Geometry check sheet. Reference: the model listing, model coordinates, mm. Face numbers are marked on the shaded views. A direction names the side the tool comes from. Give positions to 0.01 mm unless a question says otherwise; leave off trailing zeros. Loops run counter-clockwise (first coordinate to the right, second up) from the corner with the lowest first, then second, coordinate; pieces in that order, holes last. Notation, with made-up numbers: (-17, 20) -> (-8, 20) arc R24 cw to (-8, 30) -> close; hole circle Ø10 at (83, -10.75). An arc over 180 degrees is marked (long way). One line per question, with ' | ' between items.
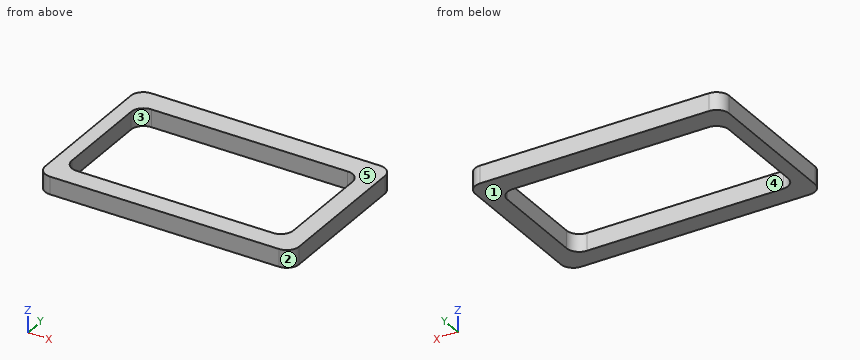
from build123d import *

# Parameters (mm, degrees)
F0_W       = 102.6703156531
F0_H       = 66.0045333207
F1_DEPTH   = 7.112
F2_W       = 89.5273201168
F2_H       = 48.7157646567
F1_FACE1_W = 102.6703156531
F1_FACE1_H = 66.0045333207
F3_DEPTH   = 7.113
F4_R       = 5.08


with BuildPart() as f1:
    # F0 (on Top) → F1 (new body)
    with BuildSketch(Plane.XY):
        with Locations((0.875947997, -11.2383794039)):
            Rectangle(F0_W, F0_H)
    extrude(amount=F1_DEPTH)

    # F2 (on face) + F1_face1 (on face) → F3 (cut, through all)
    with BuildSketch(Plane(origin=(0, 0, 0), x_dir=(1, 0, 0), z_dir=(0, 0, -1))):
        with Locations((0.0806543976, 11.7756640539)):
            Rectangle(F2_W, F2_H)
    with BuildSketch(Plane(origin=(0.875947997, -11.2383794039, 7.112), x_dir=(1, 0, 0), z_dir=(0, 0, 1))):
        Rectangle(F1_FACE1_W, F1_FACE1_H)
    extrude(amount=-F3_DEPTH, dir=(0, 0, -1), mode=Mode.SUBTRACT)

    # F4
    f4_edges = [f1.edges().sort_by_distance(p)[0] for p in [
        (-50.45921, 21.763887, 3.556),
        (52.211106, 21.763887, 3.556),
        (52.211106, -44.240646, 3.556),
        (-50.45921, -44.240646, 3.556),
        (-44.683006, -36.133546, 3.556),
        (-44.683006, 12.582218, 3.556),
        (44.844314, 12.582218, 3.556),
        (44.844314, -36.133546, 3.556),
    ]]
    fillet(f4_edges, radius=F4_R)


solid = f1.part
Item 1: Depth check by flat-ended pin: pin 1 Ø3 at (x, y) = (1.5, 9.5) entering from -Z. Enter the tip coordinate at first touch or a pass-through.
Result:
pin 1: through
Item 2: Sectioned sample at C-C (z = 2.5). Record the cut outline in (x, y), plus the area to 3 significant figures.
Result:
outline: (-50.46, -39.16) arc R5.08 ccw to (-45.38, -44.24) -> (47.13, -44.24) arc R5.08 ccw to (52.21, -39.16) -> (52.21, 16.68) arc R5.08 ccw to (47.13, 21.76) -> (-45.38, 21.76) arc R5.08 ccw to (-50.46, 16.68) -> close; hole (-44.68, -31.05) arc R5.08 ccw to (-39.6, -36.13) -> (39.76, -36.13) arc R5.08 ccw to (44.84, -31.05) -> (44.84, 7.5) arc R5.08 ccw to (39.76, 12.58) -> (-39.6, 12.58) arc R5.08 ccw to (-44.68, 7.5) -> close | area: 2,420 mm2
Item 3: Sectioned sample at A-A (y = -16). Record the cut outline in (x, z).
Result:
outline: (-50.46, 0) -> (-44.68, 0) -> (-44.68, 7.11) -> (-50.46, 7.11) -> close; (44.84, 0) -> (52.21, 0) -> (52.21, 7.11) -> (44.84, 7.11) -> close
Item 4: Sectioned sample at B-B (x = 8.5). Record the cut outline in (y, z), plus the area to 3 significant figures.
Result:
outline: (-44.24, 0) -> (-36.13, 0) -> (-36.13, 7.11) -> (-44.24, 7.11) -> close; (12.58, 0) -> (21.76, 0) -> (21.76, 7.11) -> (12.58, 7.11) -> close | area: 123 mm2
Item 5: Release check for a two-part mould opening along Y. For the marked faces 1, 2 and 3 record: pulls with the +Y half, pulls with the -Y half, needs draft (parallel to the pull), parting line crosses it, or undercut.
Result:
face 1: needs draft | face 2: pulls with the -Y half | face 3: undercut
Item 6: Scan lines: probe 1 along X at (y, z) = (-18.5, 5); probe 2 along Y at (x, z) = (39, 3.75); probe 3 along X at (y, z) = (-35.5, 0.5). Record each from-to range of solid material in increasing order.
Result:
probe 1: -50.46 to -44.68, 44.84 to 52.21 | probe 2: -44.24 to -36.13, 12.58 to 21.76 | probe 3: -50.46 to -42.06, 42.22 to 52.21
Item 7: Set-up check for the marked faces 4 and 5: record each of +Z, -Z, +X, -X, +Y, -Y from which the full face is reachable in a straight line by a thin tool's end or side.
Result:
face 4: +Z, -Z | face 5: +Z, +X, -X, +Y, -Y
